Could you check a few things on this model? Use its own coordinates, in mm. A direction names the side the tool comes from. Coordinates: 2 decimals unless noted, no trailing zeros. Loops run counter-clockwise (first coordinate to the right, second up) from the corner with the lowest first, then second, coordinate; pieces in that order, holes last. Notation, with made-up numbers: (41, -21) - (62, -21) arc R23 ccw to (62, 16) - close; hole circle Ø9 at (31, 85). An arc over 180 degrees is marked (long way). Use CSV: the item, a comma, the result in double quotes.
from build123d import *

# Parameters (mm, degrees)
SKETCH_1_W                 = 57
SKETCH_1_H                 = 45
EXTRUDE_1_DEPTH            = 3
SKETCH_2_W                 = 4
SKETCH_2_H                 = 15
EXTRUDE_2_DEPTH            = 6
SKETCH_3_W                 = 4
SKETCH_3_H                 = 15
EXTRUDE_3_DEPTH            = 6
EXTRUDE_4_DEPTH            = 3
SKETCH_5_W                 = 4
SKETCH_5_H                 = 9
EXTRUDE_5_DEPTH            = 3
CHAMFER_1_SIZE             = 3
SKETCH_6_R                 = 1.6
CUT_EXTRUDE_1_DEPTH        = 4
SKETCH_8_W                 = 8
SKETCH_8_H                 = 3
EXTRUDE_6_DEPTH            = 9
EXTRUDE_7_DEPTH            = 3
EXTRUDE_8_DEPTH            = 3
SKETCH_11_R                = 1.6
CUT_EXTRUDE_3_DEPTH        = 3
SKETCH_12_W                = 5
SKETCH_12_H                = 17
CUT_EXTRUDE_4_DEPTH        = 3
FILLET_1_R                 = 1.5
EXTRUDE_9_REACH            = 80.57
SKETCH_15_W                = 45
SKETCH_15_H                = 17.726539555
SKETCH_16_R                = 1.5
CUT_EXTRUDE_5_DEPTH        = 79.570276896
CHAMFER_1_OF_MIRROR_2_SIZE = 3


with BuildPart() as part:
    # 草图1 → 凸台-拉伸1 (new body)
    with BuildSketch(Plane(origin=(0, 0, 0), x_dir=(1, 0, 0), z_dir=(0, 1, 0))):
        with Locations((28.5, 22.5)):
            Rectangle(SKETCH_1_W, SKETCH_1_H)
    extrude(amount=EXTRUDE_1_DEPTH)

    # 草图2 → 凸台-拉伸2 (add)
    with BuildSketch(Plane.ZY):
        with Locations((-2, -1.5)):
            Rectangle(SKETCH_2_W, SKETCH_2_H)
    extrude_2 = extrude(amount=EXTRUDE_2_DEPTH)

    # 草图3 → 凸台-拉伸3 (add)
    with BuildSketch(Plane(origin=(57, 0, 0), x_dir=(0, 0, -1), z_dir=(1, 0, 0))):
        with Locations((2, -1.5)):
            Rectangle(SKETCH_3_W, SKETCH_3_H)
    extrude_3 = extrude(amount=EXTRUDE_3_DEPTH)

    # 草图4 → 凸台-拉伸4 (add)
    with BuildSketch(Plane.ZY.offset(-57)):
        Polygon((-4, -9), (-19.588457268, 0), (0, 0), (0, -9), align=None)
    extrude_4 = extrude(amount=EXTRUDE_4_DEPTH)

    # 草图5 → 凸台-拉伸5 (add)
    with BuildSketch(Plane(origin=(0, 0, 0), x_dir=(0, 0, -1), z_dir=(1, 0, 0))):
        Polygon((19.588457268, 0), (4, 0), (4, -9), align=None)
        with Locations((2, -4.5)):
            Rectangle(SKETCH_5_W, SKETCH_5_H)
    extrude_5 = extrude(amount=EXTRUDE_5_DEPTH)

    # 倒角1
    chamfer_1_edges = [part.edges().sort_by_distance(p)[0] for p in [
        (0, 3, -2),
        (57, 3, -2),
    ]]
    chamfer(chamfer_1_edges, length=CHAMFER_1_SIZE - 0.0001)  # a hair under: the kernel refuses the full size

    # 草图6 → 切除-拉伸1 (cut)
    with BuildSketch(Plane(origin=(0, 0, -4), x_dir=(-1, 0, 0), z_dir=(0, 0, -1))):
        with Locations(Location((3, -2.323268139, 0), (0, 0, 90))):
            Circle(SKETCH_6_R)
        with Locations(Location((-60, -2.323268139, 0), (0, 0, 90))):
            Circle(SKETCH_6_R)
    cut_extrude_1 = extrude(amount=-CUT_EXTRUDE_1_DEPTH, mode=Mode.SUBTRACT)

    # 草图8 → 凸台-拉伸6 (add)
    with BuildSketch(Plane.XZ):
        with Locations((28, -43.5)):
            Rectangle(SKETCH_8_W, SKETCH_8_H)
    extrude(amount=EXTRUDE_6_DEPTH)

    # 草图9 → 凸台-拉伸7 (add)
    with BuildSketch(Plane(origin=(32, 0, 0), x_dir=(0, 0, -1), z_dir=(1, 0, 0))):
        Polygon((45, 0), (29.146667939, 0), (42, -9), (45, -9), align=None)
    extrude(amount=EXTRUDE_7_DEPTH)

    # 草图10 → 凸台-拉伸8 (add)
    with BuildSketch(Plane.ZY.offset(-24)):
        Polygon((-45, 0), (-45, -9), (-42, -9), (-29.146667939, 0), align=None)
    extrude(amount=EXTRUDE_8_DEPTH)

    # 草图11 → 切除-拉伸3 (cut)
    with BuildSketch(Plane.XY.offset(-42)):
        with Locations((28, -4.5)):
            Circle(SKETCH_11_R)
    extrude(amount=-CUT_EXTRUDE_3_DEPTH, mode=Mode.SUBTRACT)

    # 草图12 → 切除-拉伸4 (cut)
    with BuildSketch(Plane(origin=(0, 3, 0), x_dir=(1, 0, 0), z_dir=(0, 1, 0))):
        with Locations((28, 19)):
            Rectangle(SKETCH_12_W, SKETCH_12_H)
    extrude(amount=-CUT_EXTRUDE_4_DEPTH, mode=Mode.SUBTRACT)

    # 圆角1
    fillet_1_edges = [part.edges().sort_by_distance(p)[0] for p in [
        (25.5, 1.5, -27.5),
        (30.5, 1.5, -27.5),
        (30.5, 1.5, -10.5),
        (25.5, 1.5, -10.5),
    ]]
    fillet(fillet_1_edges, radius=FILLET_1_R)

    # 草图15 → 凸台-拉伸9 (add, up to next)
    with BuildSketch(Plane(origin=(2.119507574, 12.02032477, 0), x_dir=(0, 0, 1), z_dir=(0.17364817766693066, 0.9848077530122081, 0)), mode=Mode.PRIVATE) as extrude_9_sk1:
        with Locations((-22.5, 43.795404353)):
            Rectangle(SKETCH_15_W, SKETCH_15_H)
    extrude_9_tool1 = extrude(extrude_9_sk1.sketch, amount=-EXTRUDE_9_REACH, mode=Mode.PRIVATE) - part.part
    extrude_9 = extrude_9_tool1.solids().sort_by_distance((45.249561, 4.415333, -22.5))[0]
    add(extrude_9)

    # 草图16 → 切除-拉伸5 (cut, through all)
    with BuildSketch(Plane(origin=(2.119507574, 12.02032477, 0), x_dir=(0.9848077530122081, -0.17364817766693064, 0), z_dir=(0.17364817766693064, 0.9848077530122081, 0))):
        with Locations(Location((43.439057305, 41, 0), (0, 0, 180))):
            Circle(SKETCH_16_R)
        with Locations((43.439057305, 4)):
            Circle(SKETCH_16_R)
    cut_extrude_5 = extrude(amount=-CUT_EXTRUDE_5_DEPTH, mode=Mode.SUBTRACT)

    # 镜向1: 凸台-拉伸9, 切除-拉伸5 across plane
    add(extrude_9.mirror(Plane(origin=(28.5, 0, 0), x_dir=(0, 0, 1), z_dir=(1, 0, 0))))
    add(cut_extrude_5.mirror(Plane(origin=(28.5, 0, 0), x_dir=(0, 0, 1), z_dir=(1, 0, 0))), mode=Mode.SUBTRACT)

    # 镜向2: 凸台-拉伸2, 凸台-拉伸3, 凸台-拉伸4, 凸台-拉伸5, 切除-拉伸1 across plane
    add(extrude_2.mirror(Plane.XY.offset(-22.5)))
    add(extrude_3.mirror(Plane.XY.offset(-22.5)))
    add(extrude_4.mirror(Plane.XY.offset(-22.5)))
    add(extrude_5.mirror(Plane.XY.offset(-22.5)))
    add(cut_extrude_1.mirror(Plane.XY.offset(-22.5)), mode=Mode.SUBTRACT)

    # 倒角1 of 镜向2
    chamfer_1_of_mirror_2_edges = [part.edges().sort_by_distance(p)[0] for p in [
        (0, 3, -43),
        (57, 3, -43),
    ]]
    chamfer(chamfer_1_of_mirror_2_edges, length=CHAMFER_1_OF_MIRROR_2_SIZE - 0.0001)  # a hair under: the kernel refuses the full size


solid = part.part
(1) Suppose I cut it at B-B (y = -7.25). State how many separate pieces and enclosed holes the cut face has, plus the area to 3 significant figures.
Computed:
separate pieces,"5"
enclosed holes,"0"
area,"237 mm²"
(2) Suppose I cut it at C-C (z = -36). Write out the boundary of the cut face in (x, y), plus the area to 3 significant figures.
Computed:
outline,"(0, -6.11) - (3, -6.11) - (3, 0) - (21, 0) - (21, -4.8) - (24, -4.8) - (24, 0) - (32, 0) - (32, -4.8) - (35, -4.8) - (35, 0) - (54, 0) - (54, -6.11) - (57, -6.11) - (57, 3) - (53.28, 3) - (36.52, 5.95) - (36, 3) - (21, 3) - (20.48, 5.95) - (3.72, 3) - (0, 3) - close"
area,"288 mm²"
(3) Which directions (+Z, -Z, +X, -X, +Y, -Y) give clear straight access to the entire face, cutting with the end or side of a thin tool? Please do faces 3 (the face through (57, 1, -23)), 4 (the face through (21, -3, -39)), 5 (the face through (24, -3, -37)), 6 (the face through (28, 2, -10.5)).
Computed:
face 3,"+X, +Y, -Y"
face 4,"+Z, -Z, -Y"
face 5,"+Z, -Y"
face 6,"+Y, -Y"
(4) Will these pins go through, and if not, where does the flat tip stop? pin 1 (4.5 mm diameter, centred on y = -6, z = -30.5, fed in from +X); pin 2 (3 mm diameter, centred on x = 22.5, z = -14.5, fed in from -Y); pin 3 (3 mm diameter, centred on y = 0.5, z = -36.5, fed in from -X); pin 4 (1 mm diameter, centred on x = 4.5, z = -34, fed in from +Y).
Computed:
pin 1,"passes through"
pin 2,"stops at y = 0"
pin 3,"stops at x = 0"
pin 4,"stops at y = 3.23"
(5) Suppose I cut it at D-D (x = 1). Write out the boundary of the cut face in (y, z), plus the area to 3 significant figures.
Computed:
outline,"(-9, -45) - (5, -45) - (5, -41) - (3, -41) - (3, -4) - (5, -4) - (5, 0) - (-9, 0) - (-9, -4) - (0, -19.59) - (0, -25.41) - (-9, -41) - close"
area,"363 mm²"
(6) Please list where these lines run through material, in increasing order: line 1 (X direction, y = -2.25, z = -37); line 2 (X direction, y = 2, z = -12); line 3 (Y direction, x = 28, z = -42.6).
Computed:
line 1,"x = 0 to 3, 21 to 24, 32 to 35, 54 to 57"
line 2,"x = 0 to 25.5, 30.5 to 57"
line 3,"y = -9 to -6.1, -2.9 to 3"
(7) Suppose I cut it at A-A (x = 60). Write out the boundary of the cut face in (y, z), plus the area to 3 significant figures.
Computed:
outline,"(-9, -45) - (-3.92, -45) - (-3.92, -41) - (-9, -41) - close; (-9, -4) - (-3.92, -4) - (-3.92, 0) - (-9, 0) - close; (-0.72, -45) - (6, -45) - (6, -41) - (-0.72, -41) - close; (-0.72, -4) - (6, -4) - (6, 0) - (-0.72, 0) - close"
area,"94.4 mm²"
(8) Thinking about a two-plate mould opening in Z: for faces 1 (the face through (13.922, 2.39, -40.549)), 2 (the face through (63, -1, -43)), which applies, +Z half, -Z half, draft (parallel to the pull), parting line (faces both ways), or undercut?
Computed:
face 1,"undercut"
face 2,"draft"
